from build123d import *

# Parameters (mm, degrees)
F0_R     = 19.05
F1_DEPTH = 38.1
F2_DEPTH = 6.35
F4_R     = 3.175
F5_DEPTH = 6.35
F6_DEPTH = 38.1


with BuildPart() as f1:
    # F0 (on Top) → F1 (new body)
    with BuildSketch(Plane.XY):
        with BuildLine():
            ThreePointArc((12.7, -21.997045), (21.997045, -12.7), (25.4, 0))
            ThreePointArc((25.4, 0), (-12.7, 21.997045), (-12.7, -21.997045))
            ThreePointArc((-12.7, -21.997045), (0, -25.4), (12.7, -21.997045))
        make_face()
        Circle(F0_R, mode=Mode.SUBTRACT)
    extrude(amount=F1_DEPTH)

    # F0 (on Top) → F2 (join)
    with BuildSketch(Plane.XY):
        with BuildLine():
            ThreePointArc((12.7, -21.997045), (21.997045, -12.7), (25.4, 0))
            ThreePointArc((25.4, 0), (-12.7, 21.997045), (-12.7, -21.997045))
            ThreePointArc((-12.7, -21.997045), (0, -25.4), (12.7, -21.997045))
        make_face()
        Circle(F0_R, mode=Mode.SUBTRACT)
        with BuildLine():
            ThreePointArc((12.7, -21.997045), (0, -25.4), (-12.7, -21.997045))
            Line((-12.7, -21.997045), (-12.7, -38.1))
            ThreePointArc((-12.7, -38.1), (-8.980256, -47.080256), (0, -50.8))
            ThreePointArc((0, -50.8), (8.980256, -47.080256), (12.7, -38.1))
            Line((12.7, -38.1), (12.7, -21.997045))
        make_face()
    extrude(amount=F2_DEPTH)

    # F4 (on offset) → F5 (join)
    with BuildSketch(Plane.XY.offset(38.1)):
        with BuildLine():
            ThreePointArc((12.7, -21.997045), (0, -25.4), (-12.7, -21.997045))
            Line((-12.7, -21.997045), (-12.7, -38.1))
            ThreePointArc((-12.7, -38.1), (-8.980256, -47.080256), (0, -50.8))
            ThreePointArc((0, -50.8), (8.980256, -47.080256), (12.7, -38.1))
            Line((12.7, -38.1), (12.7, -21.997045))
        make_face()
        with Locations((0, -38.1)):
            Circle(F4_R, mode=Mode.SUBTRACT)
        with Locations((0, -38.1)):
            Circle(F4_R)
    extrude(amount=-F5_DEPTH)

    # F4 (on offset) → F6 (join)
    with BuildSketch(Plane.XY.offset(38.1)):
        with Locations((0, -38.1)):
            Circle(F4_R)
    extrude(amount=-F6_DEPTH)


solid = f1.part
Input: part model. Units: mm. Frame: model coordinates. A direction names the side the tool comes from. Coordinates: 2 decimals unless noted, no trailing zeros. Loops run counter-clockwise (first coordinate to the right, second up) from the corner with the lowest first, then second, coordinate; pieces in that order, holes last.
Q1. Cut plane C-C (x = 14). Output: boundary loops of the cut face in (y, z).
Q2. Set-up query: faces 3 (the face through (0, -21, 38.1)), 4 (the face through (12.7, -30, 35)), 5 (the face through (-3, -36, 31.75)), 6 (the face through (-12.7, -30, 3)). Return all of +Z, -Z, +X, -X, +Y, -Y with unobstructed straight access to the full face (end or side cutting, diameter ignored); none if empty.
Q3. Cut plane B-B (z = 27). Output: boundary loops of the cut face in (x, y) (3 decimals), then the cut area to 3 significant figures.
Q4. Material intervals for line 1 (Y direction, x = 0, z = 22) (3 decimals); line 2 (Z direction, x = -2.5, y = -35); line 3 (Y direction, x = 16, z = 26), sorted ascending.
Q5. Cut plane A-A (x = -2). Output: boundary loops of the cut face in (y, z).
Q6. Contact query for flat-ended pins moving along their axis: pin 1 (3 mm diameter, centred on y = -26, z = 2, fed in from -X); pin 2 (10 mm diameter, centred on y = -41.5, z = 6, fed in from +X); pin 3 (8 mm diameter, centred on x = -11.5, y = 6, fed in from -Z); pin 4 (5 mm diameter, centred on y = -37, z = 16, fed in from +X) (3 decimals). Output: stop coordinate, or through.
Q7. Draft query along Y for faces 1 (the face through (12.7, -30, 3)), 2 (the face through (1.707, -35.423, 19.228)). Return one class per face: +Y half, -Y half, draft (parallel to the pull), parting line (faces both ways), or undercut.
Q8. Cut plane D-D (y = 5). Output: boundary loops of the cut face in (x, z).
Working result:
1. outline: (-21.19, 0) - (-12.92, 0) - (-12.92, 38.1) - (-21.19, 38.1) - close; (12.92, 0) - (21.19, 0) - (21.19, 38.1) - (12.92, 38.1) - close
2. face 3: +Z, +X, -X, +Y, -Y
2. face 4: +Z, -Z, +X, -Y
2. face 5: none
2. face 6: +Z, -Z, -X, -Y
3. outline: (-12.7, -21.997) arc R25.4 ccw to (12.7, -21.997) arc R25.4 ccw (long way) to start; circle Ø6.35 at (0, -38.1); hole circle Ø38.1 at (0, 0)
3. area: 918 mm2
4. line 1: y = -41.275 to -34.925, -25.4 to -19.05, 19.05 to 25.4
4. line 2: z = 0 to 6.35, 31.75 to 38.1
4. line 3: y = -19.73 to -10.34, 10.34 to 19.73
5. outline: (-50.64, 0) - (-18.94, 0) - (-18.94, 38.1) - (-50.64, 38.1) - (-50.64, 31.75) - (-40.57, 31.75) - (-40.57, 6.35) - (-50.64, 6.35) - close; (18.94, 0) - (25.32, 0) - (25.32, 38.1) - (18.94, 38.1) - close; hole (-35.63, 6.35) - (-25.32, 6.35) - (-25.32, 31.75) - (-35.63, 31.75) - close
6. pin 1: stops at x = -12.7
6. pin 2: stops at x = 12.7
6. pin 3: passes through
6. pin 4: stops at x = 3.175
7. face 1: draft
7. face 2: undercut
8. outline: (-24.9, 0) - (-18.38, 0) - (-18.38, 38.1) - (-24.9, 38.1) - close; (18.38, 0) - (24.9, 0) - (24.9, 38.1) - (18.38, 38.1) - close
